Input: part model. Units: mm. Frame: model coordinates. Give positions to 0.01 mm unless a question says otherwise; leave off trailing zeros. Order: outer loops, then holes, each group sorted by start corner. A loop starts at its lowest first (then second) coordinate and runs counter-clockwise, first axis right, second up. Notation, with made-up numbers: (31.5, -16) - (86.5, -16) arc R21 cw to (86.5, -12) - close; hole circle Ø5 at (56.5, 88.25). An arc over 180 degrees is marked (long way). Use a Markdown table: item, result.
Autodesk Fusion 360 part; units mm, degrees
sketch "Sketch1" plane through (0, 0, 0) normal (0, 1, 0) x (1, 0, 0)
  line L0 (-50, 0) -> (55, 0)
  line L1 (-15, -80) -> (20, -80)
  line L2 (-50, 0) -> (-15, -80)
  line L3 (20, -80) -> (55, 0)
  dimension "d2" = 105
  dimension "d3" = 35
  dimension "d4" = 35
  dimension "d5" = 80
  dimension "d6" = 50
extrude "Extrude1" add sketch "Sketch1" along normal mid plane 6
fillet "Fillet1" radius 1 4 edges at (2.5, -3, 80) (2.5, 3, 80) (-15, 0, 80) (20, 0, 80)
chamfer "Chamfer1" distance 0.5 distance2 1 4 edges at (2.5, -3, 0) (2.5, 3, 0) (-50, 0, 0) (55, 0, 0) measured on face at (-3.4792, -3, 26.3333) measured on face at (-3.4792, 3, 26.3333) measured on face at (-26.9583, 1, 52.6667) measured on face at (31.9583, -1, 52.6667)
1. Section query B-B (z = 12). Return loops of the section in (x, y), then the cut area to 3 significant figures.
Response:
| item | result |
|---|---|
| outline | (-44.75, -3) - (49.75, -3) - (49.75, 3) - (-44.75, 3) - close |
| area | 567 mm^2 |
2. Section query A-A (y = -0.75). Return loops of the section in (x, z), then the cut area to 3 significant figures.
Response:
| item | result |
|---|---|
| outline | (-49.8, 0.46) - (-49, 0) - (54, 0) - (54.8, 0.46) - (20.26, 79.4) arc R1 ccw to (19.35, 80) - (-14.35, 80) arc R1 ccw to (-15.26, 79.4) - close |
| area | 5,600 mm^2 |
3. Section query D-D (x = 39). Return loops of the section in (y, z).
Response:
| item | result |
|---|---|
| outline | (-3, 0.5) - (-2, 0) - (2, 0) - (3, 0.5) - (3, 36.57) - (-3, 36.57) - close |
4. Material intervals for line 1 along X through (y, z) = (-0.5, 26) (3 decimals); line 2 along X through (y, z) = (-2.5, 67); line 3 along Z through (x, y) = (-19, -1.5), sorted ascending.
Response:
| item | result |
|---|---|
| line 1 | x = -38.625 to 43.625 |
| line 2 | x = -20.69 to 25.69 |
| line 3 | z = 0 to 70.86 |
5. Pin query (flat end, axial travel): pin 1 (2 mm diameter, centred on y = -0.5, z = 13.5, fed in from -X). Return the tip coordinate at first contact, or that it passes through.
Response:
| item | result |
|---|---|
| pin 1 | stops at x = -44.53 |
6. Section query C-C (x = 26.5). Return loops of the section in (y, z), then the cut area to 3 significant figures.
Response:
| item | result |
|---|---|
| outline | (-3, 0.5) - (-2, 0) - (2, 0) - (3, 0.5) - (3, 65.14) - (-3, 65.14) - close |
| area | 390 mm^2 |
